```python
from build123d import *

# Parameters (mm, degrees)
SKETCH001_W         = 321.000992
SKETCH001_H         = 61.225169
PAD001_DEPTH        = 1
PAD_DEPTH           = 50
LINEARPATTERN_COUNT = 4
LINEARPATTERN_PITCH = 29.666667


with BuildPart() as part:
    # Sketch001 → Pad001 (new body)
    with BuildSketch(Plane.XZ):
        with Locations((12.393837, 25.929693)):
            Rectangle(SKETCH001_W, SKETCH001_H)
    extrude(amount=PAD001_DEPTH)

    # Sketch → Pad (join)
    with BuildSketch(Plane.XY):
        with BuildLine():
            Line((-13.439306, 0), (19.075138, 0))
            Line((19.075138, 0), (19.075138, 19.654779))
            Line((19.075138, 19.654779), (14.074553, 19.654779))
            ThreePointArc((-8.959539, 19.075142), (2.894254, 5.983074), (14.074553, 19.654779))
            Line((-13.439306, 19.075142), (-8.959539, 19.075142))
            Line((-13.439306, 0), (-13.439306, 19.075142))
        make_face()
    pad = extrude(amount=PAD_DEPTH)

    # LinearPattern: Pad ×4
    with Locations(*[(i * LINEARPATTERN_PITCH, 0, 0) for i in range(1, LINEARPATTERN_COUNT)]):
        add(pad)


solid = part.part
```
Model file for the job. Use its own axes, mm. A direction names the side the tool comes from. Coordinates: 2 decimals unless noted, no trailing zeros. Write each loop counter-clockwise with the first axis right and the second up, starting at its lowest first coordinate (ties: lowest second). Pieces come first, ordered by that corner, then holes. Notation, with made-up numbers: (-6, 73.5) - (24, 73.5) arc R11 ccw to (24, 94.5) - close; hole circle Ø3 at (-8.75, -12). An arc over 180 degrees is marked (long way). One line per question, with ' | ' between items. Start each with the question number.
Q1. Drill centre lines: line 1 (X direction, y = 18.5, z = 5.5); line 2 (X direction, y = 17, z = 7); line 3 (Y direction, x = 49.5, z = 26.5). Where is each one in solid material? Low to high. Write a range as [from, to].
Q2. Cut at A-A, the plane y = 15.75. List the corners of the cut face in (x, z), then the cut area to 3 significant figures.
Q3. 3-axis set-ups, long thin cutter, end or side, ignore diameter. For faces 4 (the face through (-13.439, 9, 25)), 5 (the face through (46, 8, 50)), 6 (the face through (46, 8, 0)): which of +Z, -Z, +X, -X, +Y, -Y reach the whole face in a straight line?
Q4. Pull direction X, two halves, no side cores. Call faces 1 (the face through (76, 19.655, 25)), 2 (the face through (108.075, 10, 25)), 3 (the face through (91.61, 5.98, 24.65)): pulls with the +X half, pulls with the -X half, needs draft (parallel to the pull), parting line crosses it, or undercut.
Q5. Cut at D-D, the plane x = -72. List the corners of the cut face in (y, z), then the cut area to 3 significant figures.
Q6. Cut at B-B, the plane z = 17. List the corners of the cut face in (x, y), then the cut area to 3 significant figures.
Q7. Pin check, flat tips, straight feed: pin 1 (0.8 mm diameter, centred on x = 79.5, z = 16, fed in from +Y); pin 2 (2 mm diameter, centred on y = 15.5, z = 23, fed in from -X); pin 3 (0.5 mm diameter, centred on y = 19.5, z = 18.5, fed in from +X). Stop position of each tip, or through.
Q8. Cut at C-C, the plane x = 84. List the corners of the cut face in (y, z), then the cut area to 3 significant figures.
Answer below:
1) line 1: [-13.44, -9.02], [14.22, 20.65], [43.89, 50.32], [73.55, 79.98], [103.22, 108.08] | line 2: [-13.44, -9.03], [14.23, 20.63], [43.9, 50.3], [73.57, 79.97], [103.23, 108.08] | line 3: [-1, 19.08]
2) outline: (-13.44, 0) - (-8.9, 0) - (-8.9, 50) - (-13.44, 50) - close; (14.1, 0) - (20.77, 0) - (20.77, 50) - (14.1, 50) - close; (43.77, 0) - (50.44, 0) - (50.44, 50) - (43.77, 50) - close; (73.43, 0) - (80.1, 0) - (80.1, 50) - (73.43, 50) - close; (103.1, 0) - (108.08, 0) - (108.08, 50) - (103.1, 50) - close | area: 1,480 mm^2
3) face 4: +Z, -Z, -X, +Y | face 5: +Z, +X, -X, +Y | face 6: -Z, +X, -X, +Y
4) face 1: needs draft | face 2: pulls with the +X half | face 3: undercut
5) outline: (-1, -4.68) - (0, -4.68) - (0, 56.54) - (-1, 56.54) - close | area: 61.2 mm^2
6) outline: (-148.11, -1) - (172.89, -1) - (172.89, 0) - (108.08, 0) - (108.08, 19.65) - (103.07, 19.65) arc R11.65 cw (long way) to (80.04, 19.08) - (78.41, 19.08) - (78.41, 19.65) - (73.41, 19.65) arc R11.65 cw (long way) to (50.37, 19.08) - (48.74, 19.08) - (48.74, 19.65) - (43.74, 19.65) arc R11.65 cw (long way) to (20.71, 19.08) - (19.08, 19.08) - (19.08, 19.65) - (14.07, 19.65) arc R11.65 cw (long way) to (-8.96, 19.08) - (-13.44, 19.08) - (-13.44, 0) - (-148.11, 0) - close | area: 1,660 mm^2
7) pin 1: y = 19.08 | pin 2: x = -13.44 | pin 3: x = 108.08
8) outline: (-1, -4.68) - (0, -4.68) - (0, 0) - (8.8, 0) - (8.8, 50) - (0, 50) - (0, 56.54) - (-1, 56.54) - close | area: 501 mm^2
